The figure shows three views and two pictorial views of one solid part (mm, origin at its lowest corner). Answer the questions. A direction names the side the tool comes from. Give positions to 0.01 mm unless a question says otherwise; leave off trailing zeros. Loops run counter-clockwise (first coordinate to the right, second up) from the corner with the lowest first, then second, coordinate; pieces in that order, holes last. Notation, with made-up numbers: (-9.75, 27) - (32.25, 27) arc R18 cw to (32.25, 34) - close; hole circle Ø6 at (45, 78). An arc over 180 degrees is marked (long way). Use CSV: the item, a comma, the result in double quotes.
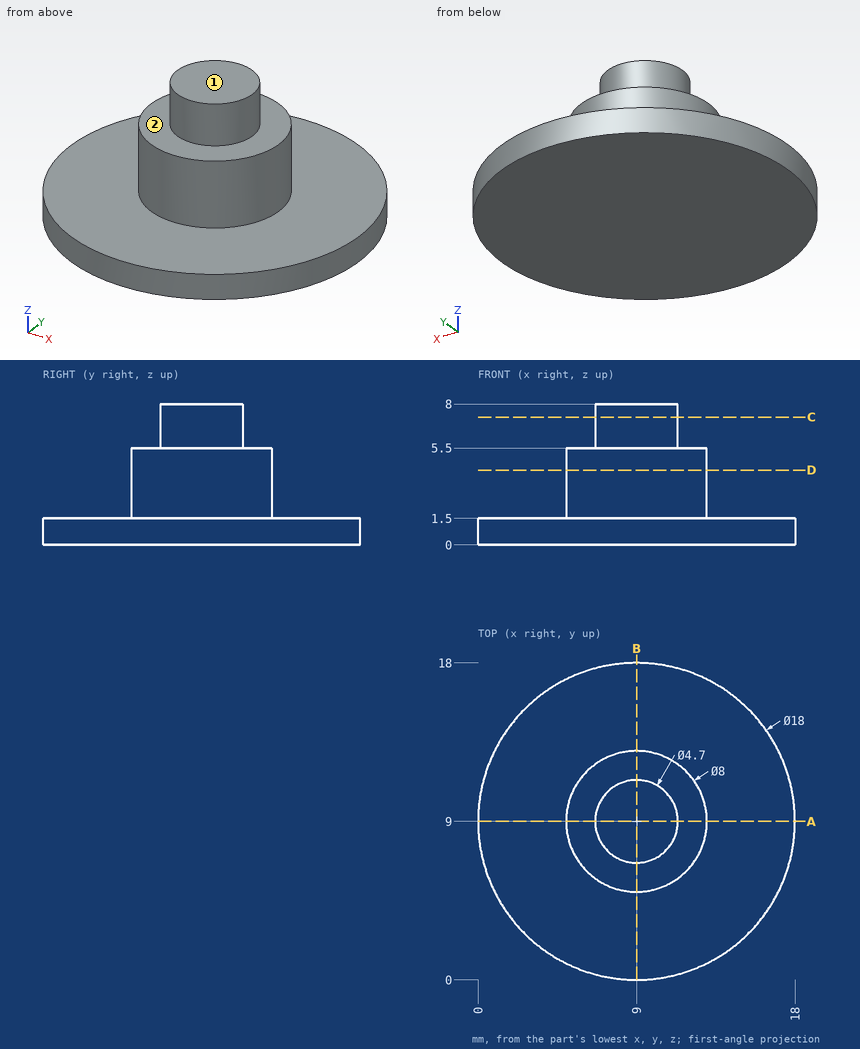
Item 1: A cutting plane is placed at C-C on z = 7.25. Determine the outline of the cut face in (x, y).
Determined:
outline,"circle Ø4.7 at (9, 9)"
Item 2: For the marked faces 1 and 2, determine the directions among +Z, -Z, +X, -X, +Y, -Y from which every point of the face is accessible in a straight line to the end or side of a thin tool.
Determined:
face 1,"+Z, +X, -X, +Y, -Y"
face 2,"+Z"
Item 3: Find the intervals of material crossed by line 1 (Z direction, x = 6, y = 15.75); line 2 (Z direction, x = 11.25, y = 7.75); line 3 (X direction, y = 7.5, z = 4.75), in increasing order.
Determined:
line 1,"z = 0 to 1.5"
line 2,"z = 0 to 5.5"
line 3,"x = 5.29 to 12.71"
Item 4: Given P1, Ø1.5, axis at x = 14, y = 3, coming from the +Z side; P2, Ø6, axis at x = 16, y = 8.5, coming from the -Z side, each flat-ended and moving along its own axis, determine where each tip first touches the part or whether it passes through.
Determined:
P1,"stops at z = 1.5"
P2,"stops at z = 0"
Item 5: A cutting plane is placed at A-A on y = 9. Determine the outline of the cut face in (x, z).
Determined:
outline,"(0, 0) - (18, 0) - (18, 1.5) - (13, 1.5) - (13, 5.5) - (11.35, 5.5) - (11.35, 8) - (6.65, 8) - (6.65, 5.5) - (5, 5.5) - (5, 1.5) - (0, 1.5) - close"
Item 6: A cutting plane is placed at D-D on z = 4.25. Determine the outline of the cut face in (x, y).
Determined:
outline,"circle Ø8 at (9, 9)"
